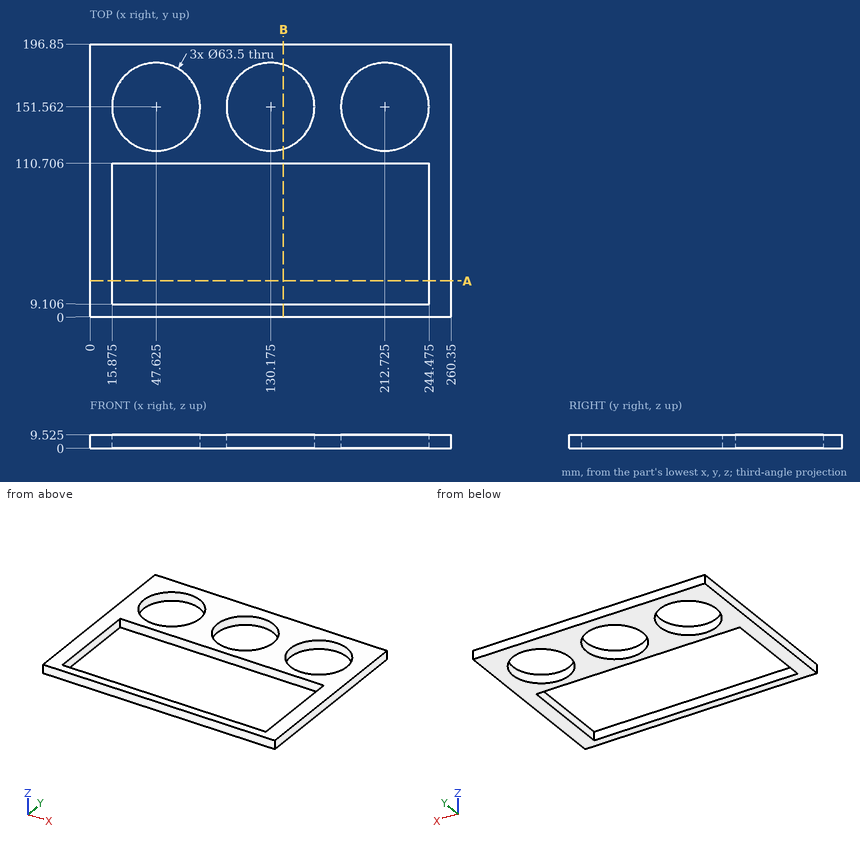
Geometry check sheet. Reference: drawing and pictorial views, mm from the part's lowest x, y, z. Round coordinates to 2 decimals unless told otherwise and drop trailing zeros. Loops run counter-clockwise (first coordinate to the right, second up) from the corner with the lowest first, then second, coordinate; pieces in that order, holes last. Notation, with made-up numbers: M 22.5,37.25 L 40.5,37.25 A17 cw 40.5,57.25 Z; hole C 63,49.25 d9. An arc over 180 degrees is marked long. Return JSON: item names as keys, results as strings. Group by question number.
(1) Section check A-A, the plane y = 26. Enter the section's corners in (x, z) (3 decimals).
(2) Scan lines: line 1 along Y through (x, z) = (130.5, 3); line 2 along X through (y, z) = (67, 9) (3 decimals); line 3 along Y through (x, z) = (59, 1.75). Record each from-to range of solid material in increasing order. Write a range as [from, to].
(3) Go/stop test with a flat-tipped pin: pin 1 (5 mm diameter, centred on x = 82.5, z = 6.5, fed in from -Y). Record where the tip stops, or that it passes through.
(4) Section check B-B, the plane x = 139.5. Give the number of separate pieces and of enclosed holes in the cut face, and give its area (3 significant figures).
Data:
{
 "1": {"outline": "M 0,0 L 15.875,0 L 15.875,9.525 L 0,9.525 Z; M 244.475,0 L 260.35,0 L 260.35,9.525 L 244.475,9.525 Z"},
 "2": {"line 1": "[0, 9.11], [110.71, 119.81], [183.31, 196.85]", "line 2": "[0, 15.875], [244.475, 260.35]", "line 3": "[0, 9.11], [110.71, 121.92], [181.2, 196.85]"},
 "3": {"pin 1": "y = 0"},
 "4": {"separate pieces": "3", "enclosed holes": "0", "area": "329 mm²"}
}
